Geometry check sheet. Reference: the model listing, model coordinates, mm. Face numbers are marked on the shaded views. A direction names the side the tool comes from. Coordinates: 2 decimals unless noted, no trailing zeros. Write each loop counter-clockwise with the first axis right and the second up, starting at its lowest first coordinate (ties: lowest second). Pieces come first, ordered by that corner, then holes. Notation, with made-up numbers: (46, -33) -> (86, -33) arc R17 cw to (86, -23) -> close; hole circle Ø4 at (-10.5, 77). An arc over 180 degrees is marked (long way). Answer in a Markdown table with one row per item. Add a question column.
Q1. Tool access check on the marked faces 5, 6 and 7. Record the directions out of +Z, -Z, +X, -X, +Y, -Y that give a thin tool (end or side, any length) a straight path to the whole face; none if there is none.
Q2. Section check B-B, the plane y = -2.5. Record the boundary of the cut face in (x, z).
Q3. Gauge pin test, flat ends, axial feed: P1, Ø1.5, axis at x = -1, y = -3, coming from the -Z side; P2, Ø2, axis at x = 3, y = -4.5, coming from the -Z side; P3, Ø1.5, axis at x = -1, z = -1, coming from the +Y side. Record the tip position at first contact, or that the pin passes through.
Q4. Release check for a two-part mould opening along X. For the marked faces 1, 2, 3 and 4 record: pulls with the +X half, pulls with the -X half, needs draft (parallel to the pull), parting line crosses it, or undercut.
Q5. Section check A-A, the plane z = 0. Record the boundary of the cut face in (x, y), and give its area (3 significant figures).
Q6. Thickness scan on line 1 (Z direction, x = 0, y = -0.45); line 2 (Z direction, x = 0, y = -1.7); line 3 (X direction, y = -4.75, z = -1.75). Record the ranges inside material, lowest first.
Q7. Section check D-D, the plane z = 1.5. Record the boundary of the cut face in (x, y).
Q8. Section check C-C, the plane x = 0. Record the boundary of the cut face in (y, z).
```python
from build123d import *

# Parameters (mm, degrees)
F0_R     = 4.06
F1_DEPTH = 5.82
F3_DEPTH = 4.06
F4_R     = 1.18
F5_DEPTH = 25
F6_R     = 2.5
F6_R_2   = 1.18
F7_DEPTH = 1.6


# Not quite as in the source:
# - a feature names something its author has since deleted; it is built from what else it names


with BuildPart() as f1:
    # F0 (on Front) → F1 (new body)
    with BuildSketch(Plane.XZ):
        Circle(F0_R)
    extrude(amount=F1_DEPTH)

    # F2 (on face) → F3 (cut)
    with BuildSketch(Plane.XZ.offset(5.82)):
        with BuildLine():
            ThreePointArc((1.6188885076, -0.61), (1.7019954639, -0.3100184526), (1.73, 0))
            ThreePointArc((1.73, 0), (1.7019954639, 0.3100184526), (1.6188885076, 0.61))
            ThreePointArc((1.6188885076, 0.61), (1.2232947315, 1.2232947315), (0.61, 1.6188885076))
            ThreePointArc((0.61, 1.6188885076), (0, 1.73), (-0.61, 1.6188885076))
            ThreePointArc((-0.61, 1.6188885076), (-1.2232947315, 1.2232947315), (-1.6188885076, 0.61))
            ThreePointArc((-1.6188885076, 0.61), (-1.73, 0), (-1.6188885076, -0.61))
            ThreePointArc((-1.6188885076, -0.61), (-1.2232947315, -1.2232947315), (-0.61, -1.6188885076))
            ThreePointArc((-0.61, -1.6188885076), (0, -1.73), (0.61, -1.6188885076))
            ThreePointArc((0.61, -1.6188885076), (1.2232947315, -1.2232947315), (1.6188885076, -0.61))
        make_face()
        with BuildLine():
            ThreePointArc((1.6188885076, 0.61), (1.7019954639, 0.3100184526), (1.73, 0))
            ThreePointArc((1.73, 0), (1.7019954639, -0.3100184526), (1.6188885076, -0.61))
            Line((1.6188885076, -0.61), (2.1288885076, -0.61))
            Line((2.1288885076, -0.61), (2.1288885076, 0.61))
            Line((2.1288885076, 0.61), (1.6188885076, 0.61))
        make_face()
        with BuildLine():
            ThreePointArc((-0.61, 1.6188885076), (0, 1.73), (0.61, 1.6188885076))
            Line((0.61, 1.6188885076), (0.61, 2.1288885076))
            Line((0.61, 2.1288885076), (-0.61, 2.1288885076))
            Line((-0.61, 2.1288885076), (-0.61, 1.6188885076))
        make_face()
        with BuildLine():
            Line((0.61, -2.1288885076), (0.61, -1.6188885076))
            ThreePointArc((0.61, -1.6188885076), (0, -1.73), (-0.61, -1.6188885076))
            Line((-0.61, -1.6188885076), (-0.61, -2.1288885076))
            Line((-0.61, -2.1288885076), (0.61, -2.1288885076))
        make_face()
        with BuildLine():
            ThreePointArc((-1.6188885076, -0.61), (-1.73, 0), (-1.6188885076, 0.61))
            Line((-1.6188885076, 0.61), (-2.1288885076, 0.61))
            Line((-2.1288885076, 0.61), (-2.1288885076, -0.61))
            Line((-2.1288885076, -0.61), (-1.6188885076, -0.61))
        make_face()
    extrude(amount=-F3_DEPTH, mode=Mode.SUBTRACT)

    # F4 (on face) → F5 (cut)
    with BuildSketch(Plane.XZ.offset(1.76)):
        Circle(F4_R)
    extrude(amount=-F5_DEPTH, mode=Mode.SUBTRACT)

    # F6 (on face) → F7 (cut)
    with BuildSketch(Plane(origin=(0, 0, 0), x_dir=(-1, 0, 0), z_dir=(0, 1, 0))):
        Circle(F6_R)
        Circle(F6_R_2, mode=Mode.SUBTRACT)
    extrude(amount=-F7_DEPTH, mode=Mode.SUBTRACT)


solid = f1.part
```
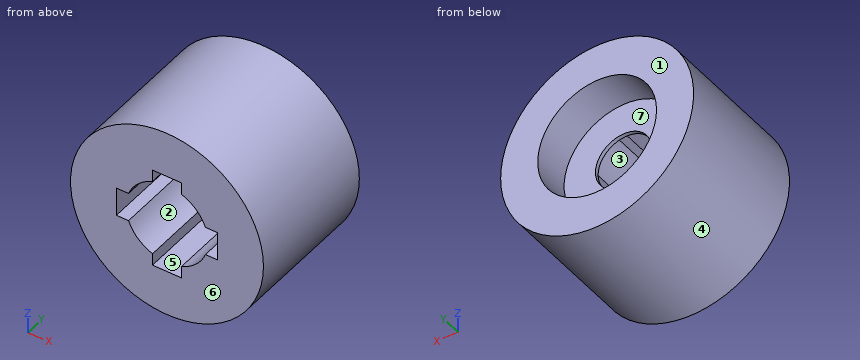
Calculated:
| question | item | result |
|---|---|---|
| 1 | face 5 | -Y |
| 1 | face 6 | +Z, -Z, +X, -X, -Y |
| 1 | face 7 | +Y |
| 2 | outline | circle Ø8.12 at (0, 0); hole (-2.13, -0.61) -> (-1.62, -0.61) arc R1.73 ccw to (-0.61, -1.62) -> (-0.61, -2.13) -> (0.61, -2.13) -> (0.61, -1.62) arc R1.73 ccw to (1.62, -0.61) -> (2.13, -0.61) -> (2.13, 0.61) -> (1.62, 0.61) arc R1.73 ccw to (0.61, 1.62) -> (0.61, 2.13) -> (-0.61, 2.13) -> (-0.61, 1.62) arc R1.73 ccw to (-1.62, 0.61) -> (-2.13, 0.61) -> close |
| 3 | P1 | stops at z = -4.05 |
| 3 | P2 | stops at z = -3.53 |
| 3 | P3 | stops at y = -1.6 |
| 4 | face 1 | needs draft |
| 4 | face 2 | undercut |
| 4 | face 3 | undercut |
| 4 | face 4 | parting line crosses it |
| 5 | outline | (-4.06, -5.82) -> (-2.13, -5.82) -> (-2.13, -1.76) -> (-1.18, -1.76) -> (-1.18, -1.6) -> (-2.5, -1.6) -> (-2.5, 0) -> (-4.06, 0) -> close; (1.18, -1.76) -> (2.13, -1.76) -> (2.13, -5.82) -> (4.06, -5.82) -> (4.06, 0) -> (2.5, 0) -> (2.5, -1.6) -> (1.18, -1.6) -> close |
| 5 | area | 21.6 mm² |
| 6 | line 1 | z = -4.06 to -2.5, 2.5 to 4.06 |
| 6 | line 2 | z = -4.06 to -1.18, 1.18 to 4.06 |
| 6 | line 3 | x = -3.66 to -0.61, 0.61 to 3.66 |
| 7 | outline | (-3.77, -5.82) -> (-0.86, -5.82) -> (-0.86, -1.76) -> (0.86, -1.76) -> (0.86, -5.82) -> (3.77, -5.82) -> (3.77, 0) -> (2, 0) -> (2, -1.6) -> (-2, -1.6) -> (-2, 0) -> (-3.77, 0) -> close |
| 8 | outline | (-5.82, -4.06) -> (0, -4.06) -> (0, -2.5) -> (-1.6, -2.5) -> (-1.6, -1.18) -> (-1.76, -1.18) -> (-1.76, -2.13) -> (-5.82, -2.13) -> close; (-5.82, 2.13) -> (-1.76, 2.13) -> (-1.76, 1.18) -> (-1.6, 1.18) -> (-1.6, 2.5) -> (0, 2.5) -> (0, 4.06) -> (-5.82, 4.06) -> close |
